The listing builds one solid part. Answer for the finished solid, in the listing's coordinates (mm). Give positions to 0.01 mm unless a question says otherwise; leave off trailing zeros. Write each loop counter-clockwise with the first axis right and the second up, starting at its lowest first coordinate (ties: lowest second). Pieces come first, ordered by that corner, then holes. Notation, with made-up numbers: M -12.75,16 L 44.25,16 A34 cw 44.25,51 Z; hole C 40,68.5 d10. An arc over 180 degrees is marked long. Return JSON: item names as keys, results as strings.
from build123d import *

# Parameters (mm, degrees)
SKETCH1_W           = 127
SKETCH1_H           = 76.2
BOSS_EXTRUDE1_DEPTH = 3.175
SKETCH3_W           = 127
SKETCH3_H           = 38.1
SKETCH3_R           = 3.25
CUT_EXTRUDE1_DEPTH  = 4.175


with BuildPart() as part:
    # Sketch1 → Boss-Extrude1 (new body)
    with BuildSketch(Plane(origin=(0, 0, 0), x_dir=(1, 0, 0), z_dir=(0, 1, 0))):
        Rectangle(SKETCH1_W, SKETCH1_H)
    extrude(amount=BOSS_EXTRUDE1_DEPTH)

    # Sketch3 → Cut-Extrude1 (cut, through all)
    with BuildSketch(Plane(origin=(0, 3.175, 0), x_dir=(1, 0, 0), z_dir=(0, 1, 0))):
        with Locations((0, -19.05)):
            Rectangle(SKETCH3_W, SKETCH3_H)
        with Locations((-53, 28.1)):
            Circle(SKETCH3_R)
        with Locations((53, 28.1)):
            Circle(SKETCH3_R)
    extrude(amount=-CUT_EXTRUDE1_DEPTH, mode=Mode.SUBTRACT)


solid = part.part
Item 1: A cutting plane is placed at B-B, the plane z = -28.1. Write down the section's boundary in (x, y) (3 decimals), plus the area to 3 significant figures.
Geometry results:
{"outline": "M -63.5,0 L -56.25,0 L -56.25,3.175 L -63.5,3.175 Z; M -49.75,0 L 49.75,0 L 49.75,3.175 L -49.75,3.175 Z; M 56.25,0 L 63.5,0 L 63.5,3.175 L 56.25,3.175 Z", "area": "362 mm2"}
Item 2: Determine the mould class of faces 1 (the cylindrical face through (-51.25, 1.61, -30.84)), 2 (the flat face through (63.5, 2, -19)), 3 (the flat face through (-1, 2, 0)), 4 (the cylindrical face through (54.75, 1.61, -30.84)) for opening direction X: +X half, -X half, draft (parallel to the pull), parting line (faces both ways), or undercut.
Geometry results:
{"face 1": "undercut", "face 2": "+X half", "face 3": "draft", "face 4": "undercut"}
Item 3: Given pin 1 Ø1 at (x, z) = (10.5, -28) entering from -Y; pin 2 Ø6 at (x, z) = (53, -28.1) entering from +Y, each flat-ended and moving along its own axis, determine where each tip first touches the part or whether it passes through.
Geometry results:
{"pin 1": "stops at y = 0", "pin 2": "passes through"}
Item 4: Find the intervals of material crossed by line 1 (X direction, y = 1.45, z = -28.1); line 2 (X direction, y = 0.85, z = -29); line 3 (Z direction, x = 53, y = 1.65), in increasing order.
Geometry results:
{"line 1": "x = -63.5 to -56.25, -49.75 to 49.75, 56.25 to 63.5", "line 2": "x = -63.5 to -56.12, -49.88 to 49.88, 56.12 to 63.5", "line 3": "z = -38.1 to -31.35, -24.85 to 0"}
Item 5: A cutting plane is placed at A-A, the plane x = -53. Write down the section's boundary in (y, z) (3 decimals).
Geometry results:
{"outline": "M 0,-38.1 L 3.175,-38.1 L 3.175,-31.35 L 0,-31.35 Z; M 0,-24.85 L 3.175,-24.85 L 3.175,0 L 0,0 Z"}
